```python
from build123d import *

# Parameters (mm, degrees)
SKETCH1_W           = 12.7
SKETCH1_H           = 101.6
BOSS_EXTRUDE1_DEPTH = 59.999999888
SKETCH2_W           = 9.525
SKETCH2_H           = 101.6
CUT_EXTRUDE1_DEPTH  = 53.65
SKETCH3_R           = 1.000000032
CUT_EXTRUDE2_DEPTH  = 7.35


with BuildPart() as part:
    # Sketch1 → Boss-Extrude1 (new body)
    with BuildSketch(Plane(origin=(0, 0, 0), x_dir=(1, 0, 0), z_dir=(0, 1, 0))):
        Rectangle(SKETCH1_W, SKETCH1_H)
    extrude(amount=BOSS_EXTRUDE1_DEPTH)

    # Sketch2 → Cut-Extrude1 (cut)
    with BuildSketch(Plane(origin=(0, 59.999999888, 0), x_dir=(1, 0, 0), z_dir=(0, 1, 0))):
        with Locations((1.5875, 0)):
            Rectangle(SKETCH2_W, SKETCH2_H)
    extrude(amount=-CUT_EXTRUDE1_DEPTH, mode=Mode.SUBTRACT)

    # Sketch3 → Cut-Extrude2 (cut, through all)
    with BuildSketch(Plane(origin=(0, 6.35, 0), x_dir=(1, 0, 0), z_dir=(0, 1, 0))):
        with Locations((0, 38.1)):
            Circle(SKETCH3_R)
        with Locations((0, 12.7)):
            Circle(SKETCH3_R)
        with Locations((0, -12.7)):
            Circle(SKETCH3_R)
        with Locations((0, -38.1)):
            Circle(SKETCH3_R)
    extrude(amount=-CUT_EXTRUDE2_DEPTH, mode=Mode.SUBTRACT)


solid = part.part
```
Can you work these out from the model? Positions are in its coordinate system, mm. A direction names the side the tool comes from. Give positions to 0.01 mm unless a question says otherwise; leave off trailing zeros. Order: outer loops, then holes, each group sorted by start corner. A loop starts at its lowest first (then second) coordinate and runs counter-clockwise, first axis right, second up. Notation, with made-up numbers: M 13.5,74.25 L 23.5,74.25 A16 cw 23.5,78.25 Z; hole C 28.25,43 d1. An arc over 180 degrees is marked long. Write item = value, one per line. Start each with the question number.
Q1. Suppose I cut it at D-D (y = 14). Write out the boundary of the cut face in (x, z) (3 decimals), plus the area to 3 significant figures.
Q2. Suppose I cut it at C-C (z = 5.5). Write out the boundary of the cut face in (x, y) (3 decimals), plus the area to 3 significant figures.
Q3. I need wall thicknesses on probe 1 along Z at (x, y) = (0, 3.75); probe 2 along X at (y, z) = (4, 38); probe 3 along Y at (x, z) = (-2, 28). Which ranges of each line are inside material? Lowest first, please. Write a range as [from, to].
Q4. Suppose I cut it at A-A (x = 0). Write out the boundary of the cut face in (y, z).
Q5. Suppose I cut it at B-B (z = -38.1). Write out the boundary of the cut face in (x, y) (3 decimals), plus the area to 3 significant figures.
Q6. Will these pins go through, and if not, where does the flat tip stop? pin 1 Ø5 at (x, z) = (1, -11) entering from +Y; pin 2 Ø10 at (y, z) = (44.5, -25.5) entering from +X (3 decimals).
Q7. For faces 1 (the flat face through (-3.175, 34, 1)), 2 (the cylindrical face through (-0.217, 3.219, 39.076)), which set-ups out of +Z, -Z, +X, -X, +Y, -Y let a thin tool reach every point of the face, with its end or its side?
Check result:
q1.outline = M -6.35,-50.8 L -3.175,-50.8 L -3.175,50.8 L -6.35,50.8 Z
q1.area = 323 mm2
q2.outline = M -6.35,0 L 6.35,0 L 6.35,6.35 L -3.175,6.35 L -3.175,60 L -6.35,60 Z
q2.area = 251 mm2
q3.probe_1 = [-50.8, -39.1], [-37.1, -13.7], [-11.7, 11.7], [13.7, 37.1], [39.1, 50.8]
q3.probe_2 = [-6.35, -0.99], [0.99, 6.35]
q3.probe_3 = [0, 6.35]
q4.outline = M 0,-50.8 L 6.35,-50.8 L 6.35,-39.1 L 0,-39.1 Z; M 0,-37.1 L 6.35,-37.1 L 6.35,-13.7 L 0,-13.7 Z; M 0,-11.7 L 6.35,-11.7 L 6.35,11.7 L 0,11.7 Z; M 0,13.7 L 6.35,13.7 L 6.35,37.1 L 0,37.1 Z; M 0,39.1 L 6.35,39.1 L 6.35,50.8 L 0,50.8 Z
q5.outline = M -6.35,0 L -1,0 L -1,6.35 L -3.175,6.35 L -3.175,60 L -6.35,60 Z; M 1,0 L 6.35,0 L 6.35,6.35 L 1,6.35 Z
q5.area = 238 mm2
q6.pin_1 = 6.35
q6.pin_2 = -3.175
q7.face_1 = +Z, -Z, +X, +Y
q7.face_2 = +Y, -Y
